```python
from build123d import *

# Parameters (mm, degrees)
ESQUISSE1_R      = 2.5
EXTRUSION1_DEPTH = 25
ESQUISSE2_W      = 30
ESQUISSE2_H      = 21
EXTRUSION2_DEPTH = 88.731584025


with BuildPart() as part:
    # Esquisse1 → Extrusion1 (new body)
    with BuildSketch(Plane(origin=(0, 0, 0), x_dir=(1, 0, 0), z_dir=(0, 1, 0))):
        with BuildLine():
            Line((0, 0), (-3, 0))
            Line((-3, 0), (-3, -80))
            Line((-3, -80), (35.567256581, -125.962666587))
            ThreePointArc((35.567256581, -125.962666587), (44.362418985, -122.157654154), (34.919767033, -120.523847112))
            Line((34.919767033, -120.523847112), (0, -78.908089297))
            Line((0, -78.908089297), (0, 0))
        make_face()
        with Locations((39.397478797, -122.748728539)):
            Circle(ESQUISSE1_R, mode=Mode.SUBTRACT)
    extrude(amount=EXTRUSION1_DEPTH)

    # Esquisse2 → Extrusion2 (cut, through all)
    with BuildSketch(Plane(origin=(-41.152782387, 0, 34.531284523), x_dir=(0.64278761, 0, 0.766044443), z_dir=(-0.766044443, 0, 0.64278761))):
        with Locations((122.35519262, 12.5)):
            Rectangle(ESQUISSE2_W, ESQUISSE2_H)
    extrude(amount=-EXTRUSION2_DEPTH, mode=Mode.SUBTRACT)


solid = part.part
```
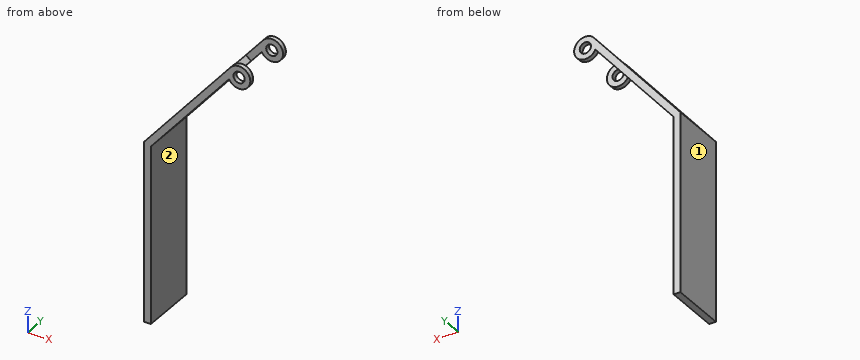
CAD build for the part. Positions are in the model's coordinates, mm. Face numbers are marked on the shaded views. Round coordinates to 2 decimals unless told otherwise and drop trailing zeros. Write each loop counter-clockwise with the first axis right and the second up, starting at its lowest first coordinate (ties: lowest second). Pieces come first, ordered by that corner, then holes. Notation, with made-up numbers: (19, -6.5) - (57, -6.5) arc R22 cw to (57, 10.5) - close; hole circle Ø1 at (5.5, 25). An arc over 180 degrees is marked (long way). Return JSON: item names as keys, results as strings. Group by question number.
Item 1: Flat gauge pins, fed straight in: pin 1 Ø4.5 at (x, z) = (39.4, 122.75) entering from -Y; pin 2 Ø6 at (y, z) = (17, 64.5) entering from +X; pin 3 Ø1 at (y, z) = (16.5, 111) entering from -X. Where does each tip first touch, or does it go through?
Item 2: Band-saw the part on A-A on x = 32. List the corners of the cut face in (y, z), plus the area to 3 significant figures.
Item 3: Band-saw the part on C-C on z = 15.5. List the corners of the cut face in (x, y).
Item 4: Band-saw the part on D-D on x = 6. List the corners of the cut face in (y, z).
Item 5: Probe probe 1 along X at (y, z) = (14, 39.5); probe 2 along Z at (x, y) = (38, 23.75); probe 3 along Z at (x, y) = (11, 7). List the from-to ranges inside material, lowest first.
Item 6: Mould opens along X. For the marked faces 1 and 2 say: +X half, -X half, draft (parallel to the pull), parting line (faces both ways), or undercut.
Item 7: Band-saw the part on B-B on y = 7. List the corners of the cut face in (x, z).
Resolved:
{
 "1": {"pin 1": "passes through", "pin 2": "stops at x = 0", "pin 3": "stops at x = 22.59"},
 "2": {"outline": "(0, 117.04) - (2, 117.04) - (2, 121.71) - (0, 121.71) - close; (23, 117.04) - (25, 117.04) - (25, 121.71) - (23, 121.71) - close", "area": "18.7 mm²"},
 "3": {"outline": "(-3, 0) - (0, 0) - (0, 25) - (-3, 25) - close"},
 "4": {"outline": "(0, 86.06) - (25, 86.06) - (25, 90.73) - (0, 90.73) - close"},
 "5": {"probe 1": "x = -3 to 0", "probe 2": "z = 117.95 to 120.68, 124.82 to 127.55", "probe 3": "z = 92.02 to 96.68"},
 "6": {"face 1": "-X half", "face 2": "+X half"},
 "7": {"outline": "(-3, 0) - (0, 0) - (0, 78.91) - (30.15, 114.84) - (27.85, 116.77) - (-3, 80) - close"}
}
